CAD build for the part. Positions are in the model's coordinates, mm. Face numbers are marked on the shaded views. A direction names the side the tool comes from. Give positions to 0.01 mm unless a question says otherwise; leave off trailing zeros. Loops run counter-clockwise (first coordinate to the right, second up) from the corner with the lowest first, then second, coordinate; pieces in that order, holes last. Notation, with made-up numbers: (41, 19) - (63, 19) arc R28 ccw to (63, 52) - close; hole circle Ø8 at (61, 2). An arc over 180 degrees is marked (long way). Return JSON: item names as keys, results as strings.
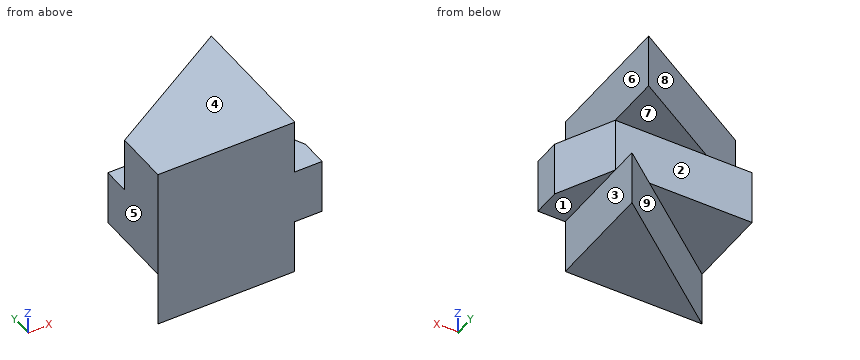
from build123d import *

# Parameters (mm, degrees)
BOSS_EXTRUDE9_DEPTH  = 10
BOSS_EXTRUDE10_DEPTH = 10
SKETCH8_W            = 25
SKETCH8_H            = 10
BOSS_EXTRUDE11_DEPTH = 10
BOSS_EXTRUDE12_DEPTH = 10


with BuildPart() as part:
    # Sketch1 → Boss-Extrude9 (new body)
    with BuildSketch(Plane.XY):
        Polygon((-25, 0), (0, 0), (0, 20), align=None)
    extrude(amount=BOSS_EXTRUDE9_DEPTH)

    # Sketch7 → Boss-Extrude10 (add)
    with BuildSketch(Plane.XY.offset(10)):
        Polygon((-25, 0), (-25, 15), (0, 15), (5, 5), (5, 0), align=None)
    extrude(amount=BOSS_EXTRUDE10_DEPTH)

    # Sketch8 → Boss-Extrude11 (add)
    with BuildSketch(Plane.XY.offset(20)):
        with Locations((-12.5, 5)):
            Rectangle(SKETCH8_W, SKETCH8_H)
    extrude(amount=BOSS_EXTRUDE11_DEPTH)

    # Sketch9 → Boss-Extrude12 (add)
    with BuildSketch(Plane.XY.offset(20)):
        Polygon((-25, 10), (0, 25), (0, 10), align=None)
    extrude(amount=BOSS_EXTRUDE12_DEPTH)


solid = part.part
1. Cut at C-C, the plane z = 23.5. Write the cut outline in (x, y), plus the area to 4 significant figures.
Values follow:
{"outline": "(-25, 0) - (0, 0) - (0, 25) - (-25, 10) - close", "area": "437.5 mm²"}
2. Drop flat-ended pins along their axis: P1, Ø4, axis at x = 2.5, y = 9.5, coming from the -Z side; P2, Ø3, axis at x = -6, y = 22, coming from the -Z side; P3, Ø8, axis at y = 12.5, z = 25.5, coming from the +X side. Give the stop position or say it passes through.
Values follow:
{"P1": "stops at z = 10", "P2": "stops at z = 20", "P3": "stops at x = 0"}
3. Pull direction Z, two halves, no side cores. Call the marked faces 1, 2, 3 and 4: +Z half, -Z half, draft (parallel to the pull), parting line (faces both ways), or undercut.
Values follow:
{"face 1": "-Z half", "face 2": "undercut", "face 3": "draft", "face 4": "+Z half"}
4. Cut at A-A, the plane x = -20.5. Write the cut outline in (y, z).
Values follow:
{"outline": "(0, 0) - (3.6, 0) - (3.6, 10) - (15, 10) - (15, 20) - (12.7, 20) - (12.7, 30) - (0, 30) - close"}
5. Drill centre lines: probe 1 along Z at (x, y) = (-2.5, 16.5); probe 2 along Y at (x, z) = (-7, 11.5); probe 3 along X at (y, z) = (6, 25.75). Where is each one in solid material? Low to high.
Values follow:
{"probe 1": "z = 0 to 10, 20 to 30", "probe 2": "y = 0 to 15", "probe 3": "x = -25 to 0"}
6. Cut at D-D, the plane x = -14.25. Write the cut outline in (y, z).
Values follow:
{"outline": "(0, 0) - (8.6, 0) - (8.6, 10) - (15, 10) - (15, 20) - (16.45, 20) - (16.45, 30) - (0, 30) - close"}
7. Cut at B-B, the plane y = 9. Write the cut outline in (x, z), plus the area to 4 significant figures.
Values follow:
{"outline": "(-25, 10) - (-13.75, 10) - (-13.75, 0) - (0, 0) - (0, 10) - (3, 10) - (3, 20) - (0, 20) - (0, 30) - (-25, 30) - close", "area": "667.5 mm²"}
8. Which spindle directions (+Z, -Z, +X, -X, +Y, -Y) get a long thin tool onto all of the face, cutting with end or side? Do the marked faces 5, 6, 7, 8 and 9. Say none if no direction does.
Values follow:
{"face 5": "+Z, -Z, -X, +Y, -Y", "face 6": "+Z, +X, +Y, -Y", "face 7": "+X, -X, +Y", "face 8": "+Z, -X, +Y", "face 9": "-Z, -X, +Y"}
